Source: CAD feature listing. Evaluate the final solid. Frame: model axes, mm. Coordinates: 2 decimals unless noted, no trailing zeros. Order: outer loops, then holes, each group sorted by start corner. A loop starts at its lowest first (then second) coordinate and runs counter-clockwise, first axis right, second up.
Item 1: Section C-C on z = -41.5. Return the cut outline in (x, y), then the cut area to 3 significant figures.
Item 2: Section D-D on y = 87.5. Return the cut outline in (x, z).
Item 3: Section A-A on z = 0. Return the cut outline in (x, y).
Item 4: Ray query, line 1 (Z direction, x = -41.25, y = 107); line 2 (Y direction, x = -39, z = 0); line 3 (Z direction, x = -42, y = 102.5). Return the intervals inside material, ascending.
Item 5: Section B-B on y = 107. Return the cut outline in (x, z).
Item 6: Contact query for flat-ended pins moving along their axis: P1, Ø9.5, axis at y = 107, z = 0, coming from the -X side; P2, Ø5, axis at y = 92, z = 2.5, coming from the +X side. Output: stop coordinate, or through.
from build123d import *

# Parameters (mm, degrees)
RESSALTO_EXTRUS_O1_DEPTH = 84.1375
CORTE_EXTRUS_O1_START    = -35
ESBO_O2_R                = 6
CORTE_EXTRUS_O1_DEPTH    = 26


with BuildPart() as part:
    # Esboço1 → Ressalto-extrusão1 (new body, symmetric)
    with BuildSketch(Plane.XY):
        Polygon((-60, 0), (60, 0), (60, 80), (30, 127), (-30, 127), (-60, 80), align=None)
    extrude(amount=RESSALTO_EXTRUS_O1_DEPTH, both=True)

    # Esboço2 → Corte-extrusão1 (cut, through all)
    with BuildSketch(Plane(origin=(0, 0, 0), x_dir=(0, 0, -1), z_dir=(1, 0, 0)).offset(CORTE_EXTRUS_O1_START)):
        with Locations((0, 107)):
            Circle(ESBO_O2_R)
    corte_extrus_o1 = extrude(amount=-CORTE_EXTRUS_O1_DEPTH, mode=Mode.SUBTRACT)

    # Espelhar1: Corte-extrusão1 across plane
    add(corte_extrus_o1.mirror(Plane(origin=(0, 0, 0), x_dir=(0, 0, 1), z_dir=(1, 0, 0))), mode=Mode.SUBTRACT)


solid = part.part
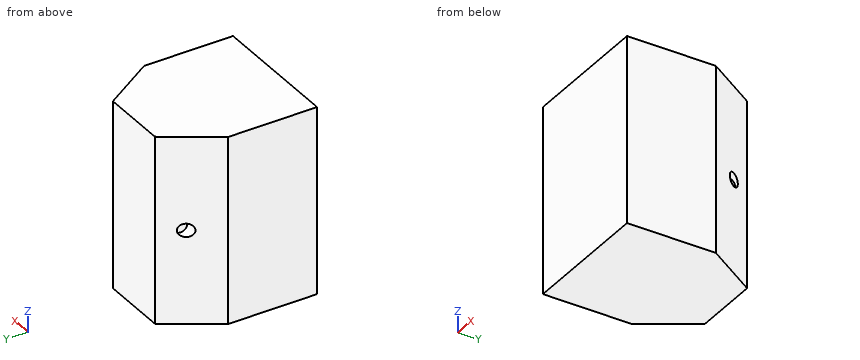
Answer list:
1. outline: (-60, 0) - (60, 0) - (60, 80) - (30, 127) - (-30, 127) - (-60, 80) - close
1. area: 13,800 mm2
2. outline: (-55.21, -84.14) - (55.21, -84.14) - (55.21, 84.14) - (-55.21, 84.14) - close
3. outline: (-60, 0) - (60, 0) - (60, 80) - (46.6, 101) - (35, 101) - (35, 113) - (38.94, 113) - (30, 127) - (-30, 127) - (-38.94, 113) - (-35, 113) - (-35, 101) - (-46.6, 101) - (-60, 80) - close
4. line 1: z = -84.14 to -6, 6 to 84.14
4. line 2: y = 0 to 101
4. line 3: z = -84.14 to -3.97, 3.97 to 84.14
5. outline: (-42.77, -84.14) - (42.77, -84.14) - (42.77, -6) - (35, -6) - (35, 6) - (42.77, 6) - (42.77, 84.14) - (-42.77, 84.14) - (-42.77, 6) - (-35, 6) - (-35, -6) - (-42.77, -6) - close
6. P1: stops at x = -35
6. P2: stops at x = 53.94
